The drawing under review shows one solid part. Ordinate dimensions are in mm from its lowest x, y, z. A direction names the side the tool comes from. Give positions to 0.01 mm unless a question says otherwise; leave off trailing zeros. Order: outer loops, then holes, each group sorted by start corner. A loop starts at its lowest first (then second) coordinate and runs counter-clockwise, first axis right, second up. Notation, with made-up numbers: (53, 45.25) - (103, 45.25) arc R21 cw to (103, 75.25) - close; hole circle Ø5 at (4, 71.25). An arc over 180 degrees is marked (long way). Write item = value, one per line. Start each with the question number.
1. We need section A-A, the plane x = 13.5. Give the boundary of the cut face in (y, z), and give its area (3 significant figures).
2. Machinability: for the marked faces 1 and 2, which of the approach directions +Z, -Z, +X, -X, +Y, -Y give a long, thin tool a straight path to every point of the face, cutting with its end or side? Answer none if there is none.
3. Wall thickness on probe 1 along Y at (x, z) = (13.5, 8.5); probe 2 along Z at (x, y) = (5.5, 2.75); probe 3 along X at (y, z) = (10.5, 5.5): over which ranges is each line inside the solid? List them lowest first.
4. We need section D-D, the plane z = 3.75. Give the boundary of the cut face in (x, y), and give its area (3 significant figures).
5. For P1, Ø5, axis at x = 9.5, z = 10.5, coming from the -Y side; P2, Ø4, axis at x = 6.5, y = 3, coming from the +Z side; P3, Ø2, axis at y = 9, z = 7.5, coming from the -X side; P4, Ø3.5, axis at x = 16, y = 14, coming from the +Z side, all flat-tipped, find the tip position at first contact; note any pin that passes through.
6. Mouldability with a two-part tool opening along Y and no side actions: class the marked faces 3, 4 and 5 as pulls with the +Y half, pulls with the -Y half, needs draft (parallel to the pull), parting line crosses it, or undercut.
7. We need section C-C, the plane z = 8.5. Give the boundary of the cut face in (x, y).
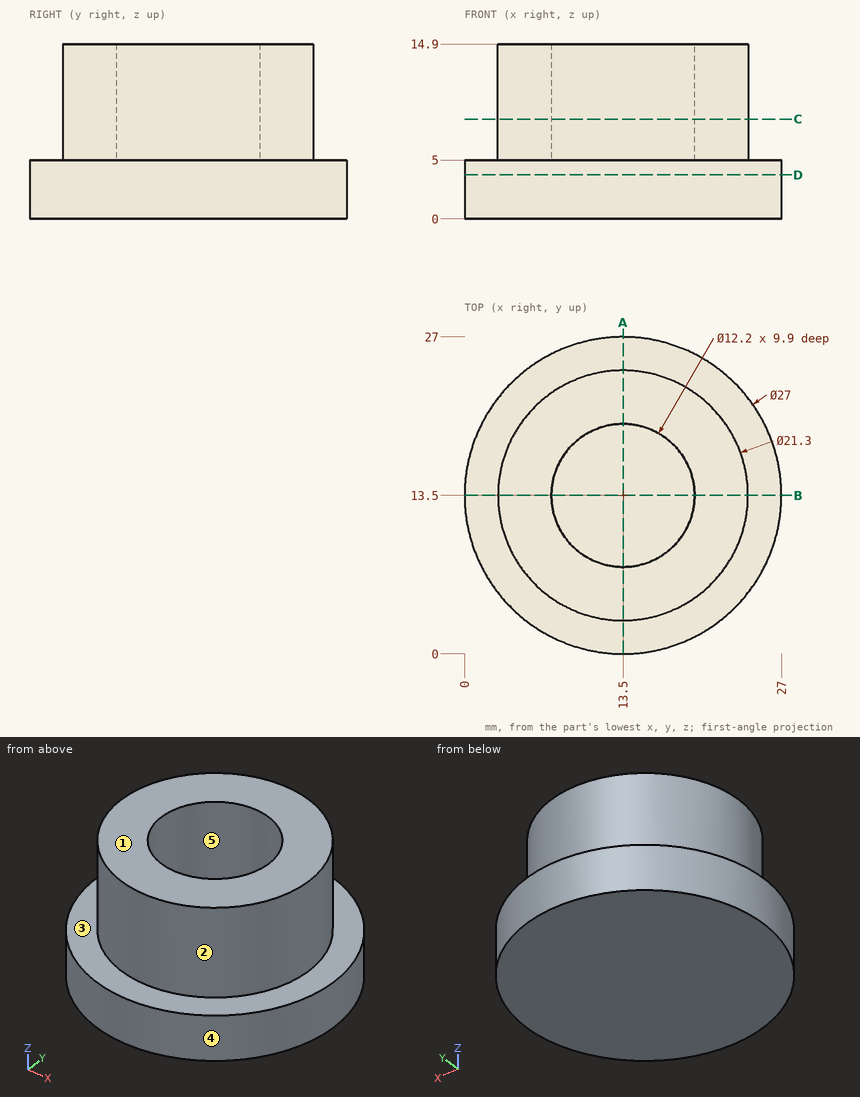
Model answer:
q1.outline = (0, 0) - (27, 0) - (27, 5) - (24.15, 5) - (24.15, 14.9) - (19.6, 14.9) - (19.6, 5) - (7.4, 5) - (7.4, 14.9) - (2.85, 14.9) - (2.85, 5) - (0, 5) - close
q1.area = 225 mm2
q2.face_1 = +Z, +X, -X, +Y, -Y
q2.face_2 = +Z
q3.probe_1 = 2.85 to 7.4, 19.6 to 24.15
q3.probe_2 = 0 to 5
q3.probe_3 = 3.28 to 8.19, 18.81 to 23.72
q4.outline = circle Ø27 at (13.5, 13.5)
q4.area = 573 mm2
q5.P1 = 2.96
q5.P2 = 14.9
q5.P3 = 3.44
q5.P4 = 5
q6.face_3 = needs draft
q6.face_4 = parting line crosses it
q6.face_5 = undercut
q7.outline = circle Ø21.3 at (13.5, 13.5); hole circle Ø12.2 at (13.5, 13.5)
